Input: part model. Units: mm. Frame: model coordinates. Coordinates: 2 decimals unless noted, no trailing zeros. Order: outer loops, then holes, each group sorted by start corner. A loop starts at its lowest first (then second) coordinate and runs counter-clockwise, first axis right, second up. Notation, with made-up numbers: (-15, 78) - (11, 78) arc R33 cw to (11, 107) - close; hole circle Ø2 at (24, 86.5). An arc over 180 degrees is marked (long way). Answer as CSV lines item,"result". Start each with the question number.
Item 1: Material intervals for line 1 along Z through (x, y) = (-5.5, 2.45); line 2 along Z through (x, y) = (50, 1.25); line 3 along Z through (x, y) = (11.5, 2.1), sorted ascending.
Item 2: Section A-A (x = -2). Output: boundary loops of the cut face in (y, z).
Item 3: Section B-B (x = -27). Output: boundary loops of the cut face in (y, z).
Item 4: Section C-C (z = 0). Output: boundary loops of the cut face in (x, y), and give its area (3 significant figures).
Item 5: First-contact query: pin 1 (2.5 mm diameter, centred on x = 35.24, z = -23.57, fed in from +Y). Flat tip, straight axial feed; report the tip coordinate or a pass-through.
Item 6: Section D-D (x = -50). Output: boundary loops of the cut face in (y, z).
from build123d import *

# Parameters (mm, degrees)
SKETCH1_W           = 160
SKETCH1_H           = 52
SKETCH1_R           = 1.5
SKETCH1_W_2         = 15
SKETCH1_H_2         = 3
BOSS_EXTRUDE1_DEPTH = 3
CUT_EXTRUDE1_DEPTH  = 3
SKETCH3_R           = 1.63582752
SKETCH3_R_2         = 1.692495787
SKETCH3_R_3         = 1.410083192
SKETCH3_R_4         = 1.550817753
CUT_EXTRUDE2_DEPTH  = 10


with BuildPart() as part:
    # Sketch1 → Boss-Extrude1 (new body)
    with BuildSketch(Plane(origin=(0, 0, 0), x_dir=(1, 0, 0), z_dir=(0, 1, 0))):
        Rectangle(SKETCH1_W, SKETCH1_H)
        with Locations((50, 10)):
            Circle(SKETCH1_R, mode=Mode.SUBTRACT)
        with Locations((60, 10)):
            Circle(SKETCH1_R, mode=Mode.SUBTRACT)
        with Locations((60, 0)):
            Circle(SKETCH1_R, mode=Mode.SUBTRACT)
        with Locations((50, 0)):
            Circle(SKETCH1_R, mode=Mode.SUBTRACT)
        with Locations((50, -10)):
            Circle(SKETCH1_R, mode=Mode.SUBTRACT)
        with Locations((60, -10)):
            Circle(SKETCH1_R, mode=Mode.SUBTRACT)
        with Locations((-60, -10)):
            Circle(SKETCH1_R, mode=Mode.SUBTRACT)
        with Locations((-50, -10)):
            Circle(SKETCH1_R, mode=Mode.SUBTRACT)
        with Locations((-50, 0)):
            Circle(SKETCH1_R, mode=Mode.SUBTRACT)
        with Locations((-60, 0)):
            Circle(SKETCH1_R, mode=Mode.SUBTRACT)
        with Locations((-60, 10)):
            Circle(SKETCH1_R, mode=Mode.SUBTRACT)
        with Locations((-50, 10)):
            Circle(SKETCH1_R, mode=Mode.SUBTRACT)
        with Locations((67.5, 14.5)):
            Rectangle(SKETCH1_W_2, SKETCH1_H_2, mode=Mode.SUBTRACT)
        with Locations((47.5, 14.5)):
            Rectangle(SKETCH1_W_2, SKETCH1_H_2, mode=Mode.SUBTRACT)
        with Locations((67.5, -14.5)):
            Rectangle(SKETCH1_W_2, SKETCH1_H_2, mode=Mode.SUBTRACT)
        with Locations((47.5, -14.5)):
            Rectangle(SKETCH1_W_2, SKETCH1_H_2, mode=Mode.SUBTRACT)
        with Locations((-47.5, -14.5)):
            Rectangle(SKETCH1_W_2, SKETCH1_H_2, mode=Mode.SUBTRACT)
        with Locations((-67.5, -14.5)):
            Rectangle(SKETCH1_W_2, SKETCH1_H_2, mode=Mode.SUBTRACT)
        with Locations((-47.5, 14.5)):
            Rectangle(SKETCH1_W_2, SKETCH1_H_2, mode=Mode.SUBTRACT)
        with Locations((-67.5, 14.5)):
            Rectangle(SKETCH1_W_2, SKETCH1_H_2, mode=Mode.SUBTRACT)
    extrude(amount=BOSS_EXTRUDE1_DEPTH)

    # Sketch2 → Cut-Extrude1 (cut)
    with BuildSketch(Plane(origin=(0, 3, 0), x_dir=(1, 0, 0), z_dir=(0, 1, 0))):
        with BuildLine():
            Line((-31.658505885, 2), (-8.266387648, 2))
            ThreePointArc((-8.266387648, 2), (-6.266387648, 0), (-8.266387648, -2))
            Line((-8.266387648, -2), (-31.658505885, -2))
            ThreePointArc((-31.658505885, -2), (-33.658505885, 0), (-31.658505885, 2))
        make_face()
        with BuildLine():
            Line((31.658505885, -9.856733432), (8.266387648, -9.856733432))
            ThreePointArc((8.266387648, -9.856733432), (6.266387648, -7.856733432), (8.266387648, -5.856733432))
            Line((8.266387648, -5.856733432), (31.658505885, -5.856733432))
            ThreePointArc((31.658505885, -5.856733432), (33.658505885, -7.856733432), (31.658505885, -9.856733432))
        make_face()
        with BuildLine():
            Line((-10.747740664, 17.987567994), (11.499478158, 17.987567994))
            ThreePointArc((11.499478158, 17.987567994), (13.499478158, 15.987567994), (11.499478158, 13.987567994))
            Line((11.499478158, 13.987567994), (-10.747740664, 13.987567994))
            ThreePointArc((-10.747740664, 13.987567994), (-12.747740664, 15.987567994), (-10.747740664, 17.987567994))
        make_face()
        with BuildLine():
            Line((-31.658505885, 9.620758334), (-8.266387648, 9.620758334))
            ThreePointArc((-8.266387648, 9.620758334), (-6.266387648, 7.620758334), (-8.266387648, 5.620758334))
            Line((-8.266387648, 5.620758334), (-31.658505885, 5.620758334))
            ThreePointArc((-31.658505885, 5.620758334), (-33.658505885, 7.620758334), (-31.658505885, 9.620758334))
        make_face()
        with BuildLine():
            Line((31.658505885, 5.620758334), (8.266387648, 5.620758334))
            ThreePointArc((8.266387648, 5.620758334), (6.266387648, 7.620758334), (8.266387648, 9.620758334))
            Line((8.266387648, 9.620758334), (31.658505885, 9.620758334))
            ThreePointArc((31.658505885, 9.620758334), (33.658505885, 7.620758334), (31.658505885, 5.620758334))
        make_face()
        with BuildLine():
            Line((-31.658505885, -5.856733432), (-8.266387648, -5.856733432))
            ThreePointArc((-8.266387648, -5.856733432), (-6.266387648, -7.856733432), (-8.266387648, -9.856733432))
            Line((-8.266387648, -9.856733432), (-31.658505885, -9.856733432))
            ThreePointArc((-31.658505885, -9.856733432), (-33.658505885, -7.856733432), (-31.658505885, -5.856733432))
        make_face()
        with BuildLine():
            Line((31.658505885, -2), (8.266387648, -2))
            ThreePointArc((8.266387648, -2), (6.266387648, 0), (8.266387648, 2))
            Line((8.266387648, 2), (31.658505885, 2))
            ThreePointArc((31.658505885, 2), (33.658505885, 0), (31.658505885, -2))
        make_face()
        with BuildLine():
            Line((-10.747740664, -13.987567994), (11.499478158, -13.987567994))
            ThreePointArc((11.499478158, -13.987567994), (13.499478158, -15.987567994), (11.499478158, -17.987567994))
            Line((11.499478158, -17.987567994), (-10.747740664, -17.987567994))
            ThreePointArc((-10.747740664, -17.987567994), (-12.747740664, -15.987567994), (-10.747740664, -13.987567994))
        make_face()
    extrude(amount=-CUT_EXTRUDE1_DEPTH, mode=Mode.SUBTRACT)

    # Sketch3 → Cut-Extrude2 (cut)
    with BuildSketch(Plane(origin=(0, 3, 0), x_dir=(1, 0, 0), z_dir=(0, 1, 0))):
        with Locations((34.323103301, -23.81549711)):
            Circle(SKETCH3_R)
        with Locations((-39.276258797, -23.81549711)):
            Circle(SKETCH3_R_2)
        with Locations((-45.484369153, 23.437784188)):
            Circle(SKETCH3_R_3)
        with Locations((35.235754497, 23.565498985)):
            Circle(SKETCH3_R_4)
    extrude(amount=-CUT_EXTRUDE2_DEPTH, mode=Mode.SUBTRACT)


solid = part.part
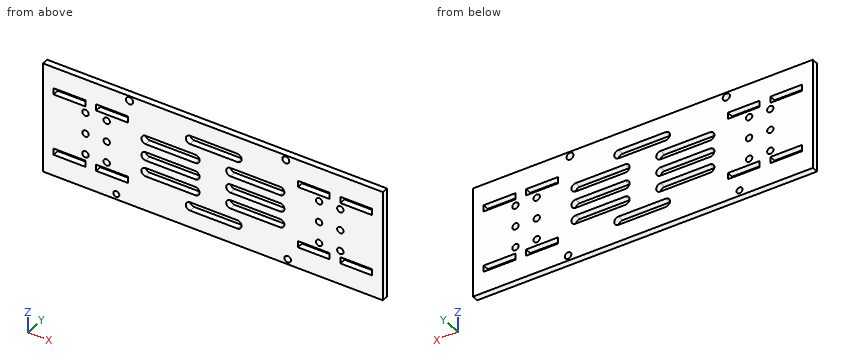
Determined:
1,line 1,"z = -26 to -17.99, -13.99 to 13.99, 17.99 to 26"
1,line 2,"z = -26 to -16, -13 to -11.5, -8.5 to -1.5, 1.5 to 8.5, 11.5 to 13, 16 to 26"
1,line 3,"z = -26 to -17.99, -13.99 to -9.62, -5.62 to -2, 2 to 5.86, 9.86 to 13.99, 17.99 to 26"
2,outline,"(0, -26) - (3, -26) - (3, -17.99) - (0, -17.99) - close; (0, -13.99) - (3, -13.99) - (3, 13.99) - (0, 13.99) - close; (0, 17.99) - (3, 17.99) - (3, 26) - (0, 26) - close"
3,outline,"(0, -26) - (3, -26) - (3, -9.62) - (0, -9.62) - close; (0, -5.62) - (3, -5.62) - (3, -2) - (0, -2) - close; (0, 2) - (3, 2) - (3, 5.86) - (0, 5.86) - close; (0, 9.86) - (3, 9.86) - (3, 26) - (0, 26) - close"
4,outline,"(-80, 0) - (-61.5, 0) - (-61.5, 3) - (-80, 3) - close; (-58.5, 0) - (-51.5, 0) - (-51.5, 3) - (-58.5, 3) - close; (-48.5, 0) - (-33.66, 0) - (-33.66, 3) - (-48.5, 3) - close; (-6.27, 0) - (6.27, 0) - (6.27, 3) - (-6.27, 3) - close; (33.66, 0) - (48.5, 0) - (48.5, 3) - (33.66, 3) - close; (51.5, 0) - (58.5, 0) - (58.5, 3) - (51.5, 3) - close; (61.5, 0) - (80, 0) - (80, 3) - (61.5, 3) - close"
4,area,"280 mm^2"
5,pin 1,"passes through"
6,outline,"(0, -26) - (3, -26) - (3, -16) - (0, -16) - close; (0, -13) - (3, -13) - (3, -11.5) - (0, -11.5) - close; (0, -8.5) - (3, -8.5) - (3, -1.5) - (0, -1.5) - close; (0, 1.5) - (3, 1.5) - (3, 8.5) - (0, 8.5) - close; (0, 11.5) - (3, 11.5) - (3, 13) - (0, 13) - close; (0, 16) - (3, 16) - (3, 26) - (0, 26) - close"
